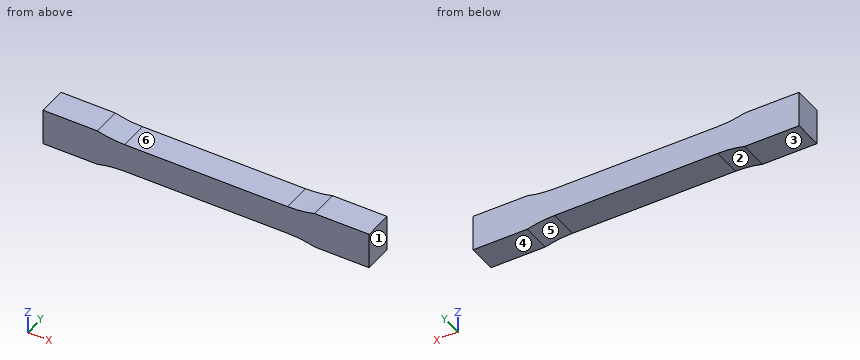
from build123d import *

# Parameters (mm, degrees)
F1_DEPTH = 20


with BuildPart() as f1:
    # F0 (on Front) → F1 (new body, symmetric)
    with BuildSketch(Plane.XZ):
        with BuildLine():
            ThreePointArc((150, 25), (131.415932, 21.255507), (112.5, 20))
            Line((112.5, 20), (0, 20))
            Line((0, 20), (-112.5, 20))
            ThreePointArc((-112.5, 20), (-131.415932, 21.255507), (-150, 25))
            Line((-150, 25), (-225, 25))
            Line((-225, 25), (-225, 0))
            Line((-225, 0), (-225, -25))
            Line((-225, -25), (-150, -25))
            ThreePointArc((-150, -25), (-131.415932, -21.255507), (-112.5, -20))
            Line((-112.5, -20), (0, -20))
            Line((0, -20), (112.5, -20))
            ThreePointArc((112.5, -20), (131.415932, -21.255507), (150, -25))
            Line((150, -25), (225, -25))
            Line((225, -25), (225, 0))
            Line((225, 0), (225, 25))
            Line((225, 25), (150, 25))
        make_face()
    extrude(amount=F1_DEPTH, both=True)


solid = f1.part
Design review of the part built by this model. Coordinates are the model's own, in mm. Face numbers are marked on the shaded views. A direction names the side the tool comes from. Give positions to 0.01 mm unless a question says otherwise; leave off trailing zeros. Order: outer loops, then holes, each group sorted by start corner. A loop starts at its lowest first (then second) coordinate and runs counter-clockwise, first axis right, second up.
1. Add section A-A, the plane y = -5. State the section outline as (x, z) points, then the cut area to 3 significant figures.
Solution:
outline: (-225, -25) - (-150, -25) arc R143.13 cw to (-112.5, -20) - (112.5, -20) arc R143.13 cw to (150, -25) - (225, -25) - (225, 25) - (150, 25) arc R143.13 cw to (112.5, 20) - (-112.5, 20) arc R143.13 cw to (-150, 25) - (-225, 25) - close
area: 19,700 mm2
2. Mouldability with a two-part tool opening along X and no side actions: class the marked faces 1, 2 and 3 as +X half, -X half, draft (parallel to the pull), parting line (faces both ways), or undercut.
Solution:
face 1: +X half
face 2: undercut
face 3: draft
3. For pin 1 Ø10 at (x, y) = (141.5, 4) entering from -Z; pin 2 Ø1 at (x, y) = (-116.5, -10.5) entering from -Z; pin 3 Ø10 at (x, y) = (66.5, 5.5) entering from +Z, all flat-tipped, find the tip position at first contact; note any pin that passes through.
Solution:
pin 1: stops at z = -24.1
pin 2: stops at z = -20.07
pin 3: stops at z = 20
4. Tool access review of the marked faces 4, 5 and 6: name each direction out of +Z, -Z, +X, -X, +Y, -Y from which nothing blocks a thin tool from reaching the whole face with its end or side.
Solution:
face 4: -Z, +X, -X, +Y, -Y
face 5: -Z, +Y, -Y
face 6: +Z, +Y, -Y
5. Add section B-B, the plane x = -66. State the section outline as (y, z) points, then the cut area to 3 significant figures.
Solution:
outline: (-20, -20) - (20, -20) - (20, 20) - (-20, 20) - close
area: 1,600 mm2
6. To check wall thickness, follow L1, parallel to Z at x = 93.5, y = -1.5; L2, parallel to Z at x = -127, y = -5. State the ranges of each line that lie inside material, in increasing order.
Solution:
L1: z = -20 to 20
L2: z = -20.74 to 20.74
